Verification items for the finished model (mm, model axes). A direction names the side the tool comes from. Give positions to 0.01 mm unless a question says otherwise; leave off trailing zeros. Loops run counter-clockwise (first coordinate to the right, second up) from the corner with the lowest first, then second, coordinate; pieces in that order, holes last. Notation, with made-up numbers: (40, 53.5) - (46, 53.5) arc R32 cw to (46, 81.5) - close; hole circle Ø10 at (57.5, -36). An arc over 180 degrees is marked (long way). Put each result on its own line as item: value. Start each with the question number.
```python
from build123d import *

# Parameters (mm, degrees)
ESTRUSIONE_ESTRUSIONE1_DEPTH = 10
SCHIZZO3_R                   = 1.62
TAGLIO_ESTRUSIONE1_DEPTH     = 8
SCHIZZO5_R                   = 1.62
TAGLIO_ESTRUSIONE4_DEPTH     = 24.5
SCHIZZO5_4_R                 = 2.5
TAGLIO_ESTRUSIONE5_DEPTH     = 24.5
SMUSSO4_SIZE                 = 1
SMUSSO5_SIZE                 = 1
SCHIZZO6_R                   = 1.62
TAGLIO_ESTRUSIONE6_DEPTH     = 24.5
SMUSSO6_SIZE                 = 1
RACCORDO1_R                  = 2


with BuildPart() as part:
    # Schizzo2 → Estrusione-Estrusione1 (new body)
    with BuildSketch(Plane.XY):
        Polygon((3, 29.438649361), (27.438649361, 5), (41.3, 5), (41.3, 0), (0, 0), (0, 5), (0, 44.039135738), (3, 44.039135738), align=None)
    extrude(amount=ESTRUSIONE_ESTRUSIONE1_DEPTH)

    # Schizzo3 → Taglio-Estrusione1 (cut)
    with BuildSketch(Plane(origin=(0, 5, 0), x_dir=(1, 0, 0), z_dir=(0, 1, 0))):
        with Locations(Location((36.62, -5.32, 0), (0, 0, 180))):
            Circle(SCHIZZO3_R)
    extrude(amount=-TAGLIO_ESTRUSIONE1_DEPTH, mode=Mode.SUBTRACT)

    # Schizzo5 → Taglio-Estrusione4 (cut)
    with BuildSketch(Plane(origin=(0, 5, 0), x_dir=(1, 0, 0), z_dir=(0, 1, 0))):
        with Locations(Location((4.68, -5.32, 0), (0, 0, 270))):
            Circle(SCHIZZO5_R)
    extrude(amount=-TAGLIO_ESTRUSIONE4_DEPTH, mode=Mode.SUBTRACT)

    # Schizzo5<4> → Taglio-Estrusione5 (cut)
    with BuildSketch(Plane(origin=(0, 5, 0), x_dir=(1, 0, 0), z_dir=(0, 1, 0))):
        with Locations(Location((4.68, -5.32, 0), (0, 0, 132.221614055))):
            Circle(SCHIZZO5_4_R)
    extrude(amount=TAGLIO_ESTRUSIONE5_DEPTH, mode=Mode.SUBTRACT)

    # Smusso4
    # the kernel refuses this chamfer: 1 mm, written as the material it takes off along each edge
    with BuildSketch(Plane(origin=(4.68, 5, 5.32), x_dir=(0, 0, 1), z_dir=(-1, 0, 0))) as smusso4_piece_1_section:
        Polygon((1.62 + SMUSSO4_SIZE, 0), (1.62, -SMUSSO4_SIZE), (1.62, 0), align=None)
    smusso4_piece_1 = revolve(axis=Axis((4.68, 5, 5.32), (0, 1, 0)), mode=Mode.PRIVATE)
    smusso4_piece_1 = smusso4_piece_1 & Plane(origin=(4.68, 4.439074745, 5.32), x_dir=(-0.6719999999981088, 0, -0.740551146108452), z_dir=(0, -1, 0)) * Cylinder(2.5, 11, mode=Mode.PRIVATE)
    add(smusso4_piece_1, mode=Mode.SUBTRACT)

    # Smusso5
    smusso5_edges = [part.edges().sort_by_distance(p)[0] for p in [
        (38.24, 5, 5.32),
    ]]
    chamfer(smusso5_edges, length=SMUSSO5_SIZE)

    # Schizzo6 → Taglio-Estrusione6 (cut)
    with BuildSketch(Plane(origin=(3, 0, 0), x_dir=(0, 0, -1), z_dir=(1, 0, 0))):
        with Locations((-5, 36.73889255)):
            Circle(SCHIZZO6_R)
    extrude(amount=-TAGLIO_ESTRUSIONE6_DEPTH, mode=Mode.SUBTRACT)

    # Smusso6
    smusso6_edges = [part.edges().sort_by_distance(p)[0] for p in [
        (3, 36.73889255, 6.62),
    ]]
    chamfer(smusso6_edges, length=SMUSSO6_SIZE)

    # Raccordo1
    raccordo1_edges = [part.edges().sort_by_distance(p)[0] for p in [
        (1.5, 44.039135738, 0),
        (41.3, 2.5, 10),
        (1.5, 44.039135738, 10),
        (41.3, 2.5, 0),
    ]]
    fillet(raccordo1_edges, radius=RACCORDO1_R)


solid = part.part
```
1) Section check D-D, the plane z = 4.25. State how many separate pieces and enclosed holes the cut face has, plus the area to 3 significant figures.
2) Draft check along Z on faces 4 (the face through (11, 12, 0)), 5 (the face through (3.694, 2.028, 4.034)), 6 (the face through (15.05, 17.39, 4.93)). Enter one of: pulls with the +Z half, pulls with the -Z half, needs draft (parallel to the pull), parting line crosses it, or undercut.
3) Section check B-B, the plane y = 18.5. Enter the section's corners in (x, z), plus the area to 3 significant figures.
4) Depth check by flat-ended pin: P1, Ø4, axis at x = 36.62, z = 5.32, coming from the +Y side; P2, Ø5, axis at x = 34, z = 6, coming from the +Y side; P3, Ø5, axis at y = 36.74, z = 5, coming from the +X side. Enter the tip coordinate at first touch or a pass-through.
5) Section check A-A, the plane x = 36.62. Enter the section's corners in (y, z).
6) Section check C-C, the plane y = 40.5. Enter the section's corners in (x, z).
7) Set-up check for faces 1 (the face through (2.216, 17.018, 5.741)), 2 (the face through (40.7, 2.46, 9.43)), 3 (the face through (3, 38.5, 2.7)): record each of +Z, -Z, +X, -X, +Y, -Y from which the full face is reachable in a straight line by a thin tool's end or side.
8) Scan lines: line 1 along Y through (x, z) = (1, 5); line 2 along X through (y, z) = (33.5, 8.5); line 3 along Z through (x, y) = (4.68, 13). Record each from-to range of solid material in increasing order. Write a range as from..to.
Results are:
1. separate pieces: 4
1. enclosed holes: 0
1. area: 483 mm2
2. face 4: pulls with the -Z half
2. face 5: undercut
2. face 6: needs draft
3. outline: (0, 0) - (13.94, 0) - (13.94, 10) - (0, 10) - close; hole circle Ø5 at (4.68, 5.32)
3. area: 120 mm2
4. P1: stops at y = 4.38
4. P2: stops at y = 5
4. P3: stops at x = 2.88
5. outline: (0, 0) - (5, 0) - (5, 2.7) - (4, 3.7) - (0, 3.7) - close; (0, 6.94) - (4, 6.94) - (5, 7.94) - (5, 10) - (0, 10) - close
6. outline: (0, 0) - (3, 0) - (3, 10) - (0, 10) - close
7. face 1: none
7. face 2: +Z, +X, +Y, -Y
7. face 3: +Z, -Z, +X, +Y
8. line 1: y = 0..35.12, 38.36..44.04
8. line 2: x = 0..3
8. line 3: z = 0..2.82, 7.82..10
